Build history of the part. All positions in model axes, mm. Face numbers are marked on the shaded views. Give positions to 0.01 mm unless a question says otherwise; leave off trailing zeros. Order: outer loops, then holes, each group sorted by start corner. A loop starts at its lowest first (then second) coordinate and runs counter-clockwise, first axis right, second up. Notation, with made-up numbers: (-13, -30) - (16, -30) arc R21 ccw to (16, -10) - close; hole circle Ø7 at (60, -9). An arc over 180 degrees is marked (long way). Use a Markdown table: item, result. Add a question column.
(1) Mould opens along Y. For the marked faces 1, 2, 3 and 4 say: +Y half, -Y half, draft (parallel to the pull), parting line (faces both ways), or undercut.
(2) Slice it at A-A (z = 4.75). Write the cut outline in (x, y), then the cut area to 3 significant figures.
(3) Flat gauge pins, fed straight in: pin 1 (1 mm diameter, centred on x = -1, z = 3, fed in from +Y); pin 2 (2 mm diameter, centred on x = -0.5, z = 4, fed in from +Y). Where does each tip first touch, or does it go through?
(4) Wall check: line 1 (X direction, y = -2, z = 1.25); line 2 (Y direction, x = 0, z = 5.25); line 3 (Y direction, x = 1, z = 3). Give the ranges that are in metal, low to high.
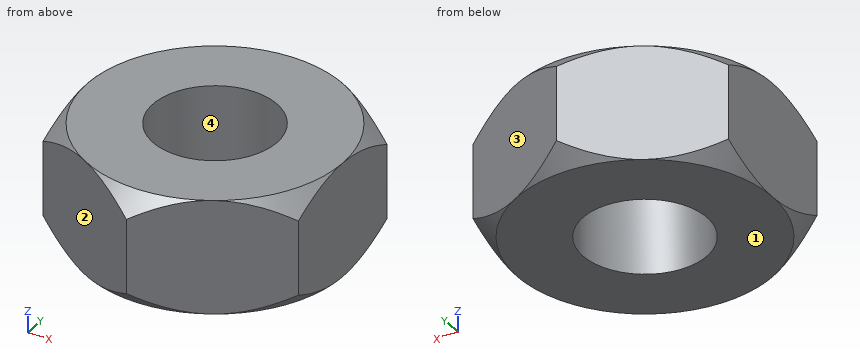
from build123d import *

# Parameters (mm, degrees)
EXTRUDE_6_DEPTH        = 6.24
HOLE_WIZARD_M8_2_D     = 6.8
HOLE_WIZARD_M8_2_DEPTH = 6.24


with BuildPart() as part:
    # 草圖12 → 填料-伸長6 (new body)
    with BuildSketch(Plane.XY):
        Polygon((7, -4.041451884), (7, 4.041451884), (0, 8.082903769), (-7, 4.041451884), (-7, -4.041451884), (0, -8.082903769), align=None)
    extrude(amount=EXTRUDE_6_DEPTH)

    # M8 螺紋孔2
    with Locations(Plane(origin=(0, 0, 0), x_dir=(-1, 0, 0), z_dir=(0, 0, -1))):
        with Locations((0, 0)):
            Hole(HOLE_WIZARD_M8_2_D / 2, depth=HOLE_WIZARD_M8_2_DEPTH)

    # 草圖17 → 除料-旋轉1 (revolve, cut)
    with BuildSketch(Plane(origin=(0, 0, 0), x_dir=(0, 0, -1), z_dir=(1, 0, 0))):
        Polygon((0, 8.082903769), (-1.082903769, 8.082903769), (0, 7), align=None)
        Polygon((-6.24, 7), (-6.24, 8.082903769), (-5.157096231, 8.082903769), align=None)
    revolve(axis=Axis((0, 0, 0), (0, 0, -1)), mode=Mode.SUBTRACT)


solid = part.part
Solution:
| question | item | result |
|---|---|---|
| 1 | face 1 | draft |
| 1 | face 2 | -Y half |
| 1 | face 3 | +Y half |
| 1 | face 4 | undercut |
| 2 | outline | (-7, -4.04) - (0, -8.08) - (7, -4.04) - (7, 4.04) - (0, 8.08) - (-7, 4.04) - close; hole circle Ø6.8 at (0, 0) |
| 2 | area | 133 mm2 |
| 3 | pin 1 | y = 7.79 |
| 3 | pin 2 | y = 8.08 |
| 4 | line 1 | -7 to -2.75, 2.75 to 7 |
| 4 | line 2 | -7.99 to -3.4, 3.4 to 7.99 |
| 4 | line 3 | -7.51 to -3.25, 3.25 to 7.51 |
